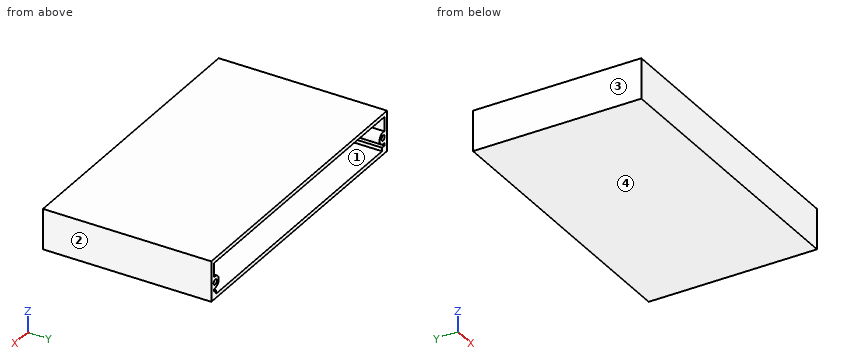
from build123d import *

# Parameters (mm, degrees)
SKETCH1_W           = 228.6
SKETCH1_H           = 31.75
BOSS_EXTRUDE1_DEPTH = 132.08
SKETCH2_W           = 222.25
SKETCH2_H           = 25.4
CUT_EXTRUDE1_DEPTH  = 128.905
SKETCH3_W           = 3.216999687
SKETCH3_H           = 4.15103562
SKETCH3_H_2         = 5.08
BOSS_EXTRUDE2_DEPTH = 128.905
SKETCH4_R           = 4.572
BOSS_EXTRUDE3_DEPTH = 128.905
SKETCH5_R           = 2.032
CUT_EXTRUDE2_DEPTH  = 123.825


with BuildPart() as part:
    # Sketch1 → Boss-Extrude1 (new body)
    with BuildSketch(Plane(origin=(0, 0, 0), x_dir=(1, 0, 0), z_dir=(0, 1, 0))):
        with Locations((114.3, 15.875)):
            Rectangle(SKETCH1_W, SKETCH1_H)
    extrude(amount=BOSS_EXTRUDE1_DEPTH)

    # Sketch2 → Cut-Extrude1 (cut)
    with BuildSketch(Plane(origin=(0, 132.08, 0), x_dir=(1, 0, 0), z_dir=(0, 1, 0))):
        with Locations((114.3, 15.875)):
            Rectangle(SKETCH2_W, SKETCH2_H)
    extrude(amount=-CUT_EXTRUDE1_DEPTH, mode=Mode.SUBTRACT)

    # Sketch3 → Boss-Extrude2 (add)
    with BuildSketch(Plane(origin=(0, 3.175, 0), x_dir=(1, 0, 0), z_dir=(0, 1, 0))):
        with Locations((4.783499844, 27.85651781)):
            Rectangle(SKETCH3_W, SKETCH3_H)
        with Locations((4.783499844, 20.955)):
            Rectangle(SKETCH3_W, SKETCH3_H_2)
    boss_extrude2 = extrude(amount=BOSS_EXTRUDE2_DEPTH)

    # Mirror1: Boss-Extrude2 across plane
    add(boss_extrude2.mirror(Plane.ZY.offset(-114.3)))

    # Sketch4 → Boss-Extrude3 (add)
    with BuildSketch(Plane(origin=(0, 3.175, 0), x_dir=(1, 0, 0), z_dir=(0, 1, 0))):
        with Locations((5.08, 18.796)):
            Circle(SKETCH4_R)
        with Locations((223.52, 18.796)):
            Circle(SKETCH4_R)
    extrude(amount=BOSS_EXTRUDE3_DEPTH)

    # Sketch5 → Cut-Extrude2 (cut)
    with BuildSketch(Plane(origin=(0, 132.08, 0), x_dir=(1, 0, 0), z_dir=(0, 1, 0))):
        with Locations((5.08, 18.796)):
            Circle(SKETCH5_R)
        with Locations((223.52, 18.796)):
            Circle(SKETCH5_R)
    extrude(amount=-CUT_EXTRUDE2_DEPTH, mode=Mode.SUBTRACT)


solid = part.part
Geometry: final body of the model. Coordinates: model frame, mm. Face numbers are marked on the shaded views. Give positions to 0.01 mm unless a question says otherwise; leave off trailing zeros. Loops run counter-clockwise (first coordinate to the right, second up) from the corner with the lowest first, then second, coordinate; pieces in that order, holes last. Notation, with made-up numbers: (72, 55) -> (104, 55) arc R14 ccw to (104, 59) -> close; hole circle Ø5 at (13, -24.75). An arc over 180 degrees is marked (long way). Put each result on its own line as item: value.
1. Cut plane A-A (x = 75.5). Return the cut outline in (y, z) (3 decimals).
Taken from the geometry:
outline: (0, -31.75) -> (132.08, -31.75) -> (132.08, -28.575) -> (3.175, -28.575) -> (3.175, -3.175) -> (132.08, -3.175) -> (132.08, 0) -> (0, 0) -> close
2. Pull-direction query (X, two-part tool) for the marked faces 1, 2, 3 and 4; classes: released by +X, released by -X, zero draft, split by the parting line, or undercut.
Taken from the geometry:
face 1: undercut
face 2: released by +X
face 3: released by -X
face 4: zero draft
3. Cut plane B-B (z = -10). Return the cut outline in (x, y) (3 decimals).
Taken from the geometry:
outline: (0, 0) -> (228.6, 0) -> (228.6, 132.08) -> (225.425, 132.08) -> (225.425, 3.175) -> (3.175, 3.175) -> (3.175, 132.08) -> (0, 132.08) -> close
4. Ray query, line 1 along Z through (x, y) = (142.5, 13) (3 decimals); line 2 along Z through (x, y) = (223.52, 89.5) (3 decimals); line 3 along X through (y, z) = (9.5, -8.5) (3 decimals). Return the intervals inside material, ascending. Write a range as [from, to].
Taken from the geometry:
line 1: z = [-31.75, -28.575], [-3.175, 0]
line 2: z = [-31.75, -25.781], [-23.495, -20.828], [-16.764, -14.224], [-3.175, 0]
line 3: x = [0, 3.175], [225.425, 228.6]
5. Pin query (flat end, axial travel): P1, Ø3.5, axis at x = 5.08, z = -18.796, coming from the +Y side (3 decimals); P2, Ø7.5, axis at x = 86, z = -15.5, coming from the +Y side (3 decimals). Return the tip coordinate at first contact, or that it passes through.
Taken from the geometry:
P1: stops at y = 8.255
P2: stops at y = 3.175
6. Cut plane C-C (y = 123). Return the cut outline in (x, z) (3 decimals).
Taken from the geometry:
outline: (0, -31.75) -> (228.6, -31.75) -> (228.6, 0) -> (0, 0) -> close; hole circle Ø4.064 at (5.08, -18.796); hole (3.175, -25.781) -> (6.392, -25.781) -> (6.392, -28.575) -> (222.208, -28.575) -> (222.208, -25.781) -> (225.425, -25.781) -> (225.425, -23.495) -> (222.208, -23.495) -> (222.208, -23.176) arc R4.572 cw (long way) to (225.425, -14.64) -> (225.425, -3.175) -> (3.175, -3.175) -> (3.175, -14.64) arc R4.572 cw (long way) to (6.392, -23.176) -> (6.392, -23.495) -> (3.175, -23.495) -> close; hole circle Ø4.064 at (223.52, -18.796)
